Can you work these out from the drawing? Everything is in mm from the part's minimum corner. A direction names the side the tool comes from. Round coordinates to 2 decimals unless told otherwise and drop trailing zeros. Loops run counter-clockwise (first coordinate to the right, second up) from the corner with the lowest first, then second, coordinate; pieces in that order, holes last. Notation, with made-up numbers: (-40, 89) -> (6, 89) arc R14 ccw to (6, 95) -> close; hole circle Ø9 at (-15, 12). An arc over 180 degrees is marked (long way). One line per item, written item: value.
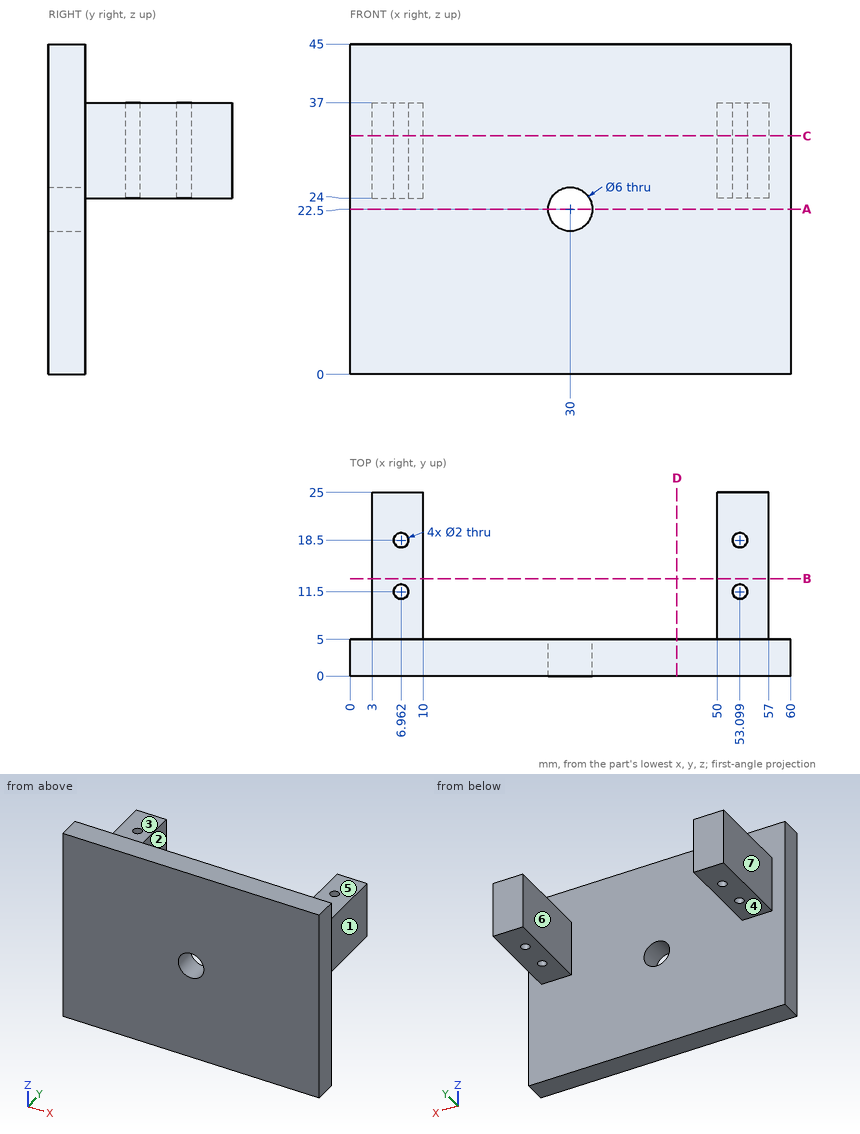
(1) Imagine slicing it at D-D on x = 44.5. Write out the boundary of the cut face in (y, z), then the cut area to 3 significant figures.
Results below:
outline: (0, 0) -> (5, 0) -> (5, 45) -> (0, 45) -> close
area: 225 mm²
(2) Imagine slicing it at C-C on z = 32.5. Write out the boundary of the cut face in (x, y).
Results below:
outline: (0, 0) -> (60, 0) -> (60, 5) -> (57, 5) -> (57, 25) -> (50, 25) -> (50, 5) -> (10, 5) -> (10, 25) -> (3, 25) -> (3, 5) -> (0, 5) -> close; hole circle Ø2 at (6.96, 11.5); hole circle Ø2 at (6.96, 18.5); hole circle Ø2 at (53.1, 11.5); hole circle Ø2 at (53.1, 18.5)
(3) We'd pull the mould along X, two halves only. Please class the marked faces 5, 6 and 7: +X half, -X half, draft (parallel to the pull), parting line (faces both ways), or undercut.
Results below:
face 5: draft
face 6: undercut
face 7: -X half
(4) On a 3-axis mill with a long thin cutter (end or side, diameter ignored), from which of +Z, -Z, +X, -X, +Y, -Y can I reach the whole of each face in a straight line? I mean the marked faces 1, 2, 3 and 4. Say none if no direction works.
Results below:
face 1: +Z, -Z, +X, +Y
face 2: +Z, -Z, +Y
face 3: +Z, +X, -X, +Y
face 4: -Z, +X, -X, +Y
(5) For pin 1 Ø2.5 at (x, y) = (53.1, 11.5) entering from +Z; pin 2 Ø6.5 at (y, z) = (20, 28) entering from +X; pin 3 Ø2 at (x, y) = (52.5, 11) entering from -Z; pin 4 Ø3 at (y, z) = (21, 21) entering from -X, each with a flat end and sliding along its axis, tell me the tip position at first contact or that it passes through.
Results below:
pin 1: stops at z = 37
pin 2: stops at x = 57
pin 3: stops at z = 24
pin 4: passes through
(6) Please list where these lines run through material, in increasing order: L1, parallel to X at y = 11.5, z = 31.5; L2, parallel to X at y = 2.9, z = 22.5; L3, parallel to Z at x = 30, y = 1.7.
Results below:
L1: x = 3 to 5.96, 7.96 to 10, 50 to 52.1, 54.1 to 57
L2: x = 0 to 27, 33 to 60
L3: z = 0 to 19.5, 25.5 to 45
(7) Imagine slicing it at A-A on z = 22.5. Write out the boundary of the cut face in (x, y).
Results below:
outline: (0, 0) -> (27, 0) -> (27, 5) -> (0, 5) -> close; (33, 0) -> (60, 0) -> (60, 5) -> (33, 5) -> close
(8) Imagine slicing it at B-B on y = 13.25. Write out the boundary of the cut face in (x, z).
Results below:
outline: (3, 24) -> (10, 24) -> (10, 37) -> (3, 37) -> close; (50, 24) -> (57, 24) -> (57, 37) -> (50, 37) -> close
